Build history of the part. All positions in model axes, mm. A direction names the side the tool comes from. Give positions to 0.01 mm unless a question says otherwise; leave off trailing zeros. Order: outer loops, then holes, each group sorted by start corner. A loop starts at its lowest first (then second) coordinate and runs counter-clockwise, first axis right, second up. Notation, with made-up numbers: M 6.5,22 L 64.5,22 A16 ccw 64.5,29 Z; hole C -27,49.5 d6. An arc over 180 degrees is marked long. One line per item, written item: value. Start each with the question number.
from build123d import *

# Parameters (mm, degrees)
SALIENTE_EXTRUIR1_DEPTH = 3
CORTAR_EXTRUIR1_DEPTH   = 3
REDONDEO1_R             = 4


with BuildPart() as part:
    # Croquis1 → Saliente-Extruir1 (new body)
    with BuildSketch(Plane.XY):
        with BuildLine():
            Line((0, 0), (0, -3))
            Line((0, -3), (-5, -3))
            Line((-5, -3), (-5, 0))
            Line((-5, 0), (-7.5, 0))
            ThreePointArc((-7.5, 0), (-20.567061666, 27.319617989), (-50.38, 22))
            Line((-50.38, 22), (-55.38, 22))
            Line((-55.38, 22), (-55.38, 20.5))
            Line((-55.38, 20.5), (-60.38, 20.5))
            Line((-60.38, 20.5), (-60.38, 22))
            Line((-60.38, 22), (-62.38, 22))
            Line((-62.38, 22), (-62.38, 58))
            Line((-62.38, 58), (-55.38, 58))
            Line((-55.38, 58), (-55.38, 61))
            Line((-55.38, 61), (-45.38, 61))
            Line((-45.38, 61), (-45.38, 58))
            Line((-45.38, 58), (-35.38, 58))
            Line((-35.38, 58), (-35.38, 61))
            Line((-35.38, 61), (-25.38, 61))
            Line((-25.38, 61), (-25.38, 58))
            Line((-25.38, 58), (-15.38, 58))
            Line((-15.38, 58), (-15.38, 61))
            Line((-15.38, 61), (-5.38, 61))
            Line((-5.38, 61), (-5.38, 58))
            Line((-5.38, 58), (2, 58))
            Line((2, 58), (2, 0))
            Line((2, 0), (0, 0))
        make_face()
    extrude(amount=SALIENTE_EXTRUIR1_DEPTH)

    # Croquis2 → Cortar-Extruir1 (cut)
    with BuildSketch(Plane.XY.offset(3)):
        with BuildLine():
            Line((-62.38, 46), (-62.38, 26))
            ThreePointArc((-62.38, 26), (-52.38, 36), (-62.38, 46))
        make_face()
    extrude(amount=-CORTAR_EXTRUIR1_DEPTH, mode=Mode.SUBTRACT)

    # Redondeo1
    redondeo1_edges = [part.edges().sort_by_distance(p)[0] for p in [
        (-62.38, 46, 1.5),
        (-62.38, 26, 1.5),
    ]]
    fillet(redondeo1_edges, radius=REDONDEO1_R)


solid = part.part
1) Slice it at C-C (x = -27.5). List the corners of the cut face in (y, z), plus the area to 3 significant figures.
2) Slice it at B-B (x = -58). List the corners of the cut face in (y, z), plus the area to 3 significant figures.
3) Pull direction X, two halves, no side cores. Call faces 1 (the flat face through (-25.38, 60, 1)), 2 (the flat face through (-10, 61, 1)), 3 (the flat face through (-5, -2, 1)): pulls with the +X half, pulls with the -X half, needs draft (parallel to the pull), parting line crosses it, or undercut.
4) Tool access for faces 4 (the flat face through (0, -1, 1)), 5 (the flat face through (-35.38, 59, 1)), 6 (the flat face through (-61, 22, 1)): list every direction of +Z, -Z, +X, -X, +Y, -Y with a clear straight run to the whole face (end or side of a thin tool).
5) Slice it at D-D (y = 33). List the corners of the cut face in (x, z), plus the area to 3 significant figures.
6) Drop flat-ended pins along their axis: P1, Ø0.9, axis at y = 59.5, z = 1, coming from the -X side; P2, Ø1.5, axis at x = -58, z = 1.5, coming from the +Y side; P3, Ø1.5, axis at y = -1, z = 2, coming from the -X side. Give the stop position or say it passes through.
7) Drill centre lines: line 1 (X direction, y = 58.5, z = 1.9); line 2 (X direction, y = 36, z = 0.8); line 3 (Y direction, x = -51.5, z = 2.6). Where is each one in solid material? Low to high.
Results list:
1. outline: M 29.67,0 L 61,0 L 61,3 L 29.67,3 Z
1. area: 94.0 mm²
2. outline: M 20.5,0 L 27.01,0 L 27.01,3 L 20.5,3 Z; M 44.99,0 L 58,0 L 58,3 L 44.99,3 Z
2. area: 58.6 mm²
3. face 1: undercut
3. face 2: needs draft
3. face 3: pulls with the -X half
4. face 4: +Z, -Z, +X, -Y
4. face 5: +Z, -Z, +Y
4. face 6: +Z, -Z, -X, -Y
5. outline: M -52.84,0 L 2,0 L 2,3 L -52.84,3 Z
5. area: 165 mm²
6. P1: stops at x = -55.38
6. P2: stops at y = 58
6. P3: stops at x = -5
7. line 1: x = -55.38 to -45.38, -35.38 to -25.38, -15.38 to -5.38
7. line 2: x = -52.38 to 2
7. line 3: y = 22 to 61
